For this review, take the finished solid that the model builds, in its own axes (mm). Face numbers are marked on the shaded views. A direction names the side the tool comes from. Coordinates: 2 decimals unless noted, no trailing zeros. Order: outer loops, then holes, each group sorted by start corner. A loop starts at its lowest first (then second) coordinate and runs counter-clockwise, first axis right, second up. Notation, with made-up numbers: M -2,53.5 L 30,53.5 A12 ccw 30,65.5 Z; hole C 57.5,-29 d6. An arc over 180 degrees is marked long. Use CSV: the item, a comma, the result in double quotes.
```python
from build123d import *

# Parameters (mm, degrees)
SKETCH1_W                       = 40
SKETCH1_H                       = 35
BOSS_EXTRUDE1_DEPTH             = 20
TAP_DRILL_FOR_M3X0_5_TAP1_D     = 2.5
TAP_DRILL_FOR_M3X0_5_TAP1_DEPTH = 4
F_8_4_8_4_DIAMETER_HOLE2_D      = 8.4
F_8_4_8_4_DIAMETER_HOLE2_DEPTH  = 15
F_8_4_8_4_DIAMETER_HOLE2_TIP    = 2.5236146
F_8_4_8_4_DIAMETER_HOLE1_D      = 8.4
F_8_4_8_4_DIAMETER_HOLE1_DEPTH  = 35
F_8_4_8_4_DIAMETER_HOLE1_TIP    = 2.5236146
F_7_0_7_DIAMETER_HOLE1_D        = 7
F_7_0_7_DIAMETER_HOLE1_DEPTH    = 15
F_7_0_7_DIAMETER_HOLE1_TIP      = 2.103012167
F_8_0_8_DIAMETER_HOLE1_D        = 8
F_8_0_8_DIAMETER_HOLE1_DEPTH    = 5.5
TAP_DRILL_FOR_M3X0_5_TAP2_D     = 2.5
TAP_DRILL_FOR_M3X0_5_TAP2_DEPTH = 5.5
CHAMFER1_SIZE                   = 0.5
G1_8_TAPPED_HOLE1_D             = 8.8
G1_8_TAPPED_HOLE1_DEPTH         = 10


with BuildPart() as part:
    # Sketch1 → Boss-Extrude1 (new body)
    with BuildSketch(Plane(origin=(0, 0, 0), x_dir=(1, 0, 0), z_dir=(0, 1, 0))):
        Rectangle(SKETCH1_W, SKETCH1_H)
    extrude(amount=BOSS_EXTRUDE1_DEPTH)

    # Tap Drill for M3x0.5 Tap1
    with Locations(Plane(origin=(0, 20, 0), x_dir=(1, 0, 0), z_dir=(0, 1, 0))):
        with Locations((-17, 14.5), (17, 14.5), (17, -14.5), (-17, -14.5)):
            Hole(TAP_DRILL_FOR_M3X0_5_TAP1_D / 2, depth=TAP_DRILL_FOR_M3X0_5_TAP1_DEPTH)

    # Ø8.4 (8.4) Diameter Hole2
    with Locations(Plane(origin=(0, 20, 0), x_dir=(1, 0, 0), z_dir=(0, 1, 0))):
        with Locations((-10, 0), (10, 0)):
            Hole(F_8_4_8_4_DIAMETER_HOLE2_D / 2, depth=F_8_4_8_4_DIAMETER_HOLE2_DEPTH)
            with Locations((0, 0, -(F_8_4_8_4_DIAMETER_HOLE2_DEPTH + F_8_4_8_4_DIAMETER_HOLE2_TIP / 2))):  # 118° drill point
                Cone(0, F_8_4_8_4_DIAMETER_HOLE2_D / 2, F_8_4_8_4_DIAMETER_HOLE2_TIP, mode=Mode.SUBTRACT)

    # Ø8.4 (8.4) Diameter Hole1
    with Locations(Plane.ZY.offset(20)):
        with Locations((0, 5)):
            Hole(F_8_4_8_4_DIAMETER_HOLE1_D / 2, depth=F_8_4_8_4_DIAMETER_HOLE1_DEPTH)
            with Locations((0, 0, -(F_8_4_8_4_DIAMETER_HOLE1_DEPTH + F_8_4_8_4_DIAMETER_HOLE1_TIP / 2))):  # 118° drill point
                Cone(0, F_8_4_8_4_DIAMETER_HOLE1_D / 2, F_8_4_8_4_DIAMETER_HOLE1_TIP, mode=Mode.SUBTRACT)

    # Ø7.0 (7) Diameter Hole1
    with Locations(Plane(origin=(0, 0, 0), x_dir=(-1, 0, 0), z_dir=(0, -1, 0))):
        with Locations((10, -10), (-10, -10), (-10, 10), (10, 10)):
            Hole(F_7_0_7_DIAMETER_HOLE1_D / 2, depth=F_7_0_7_DIAMETER_HOLE1_DEPTH)
            with Locations((0, 0, -(F_7_0_7_DIAMETER_HOLE1_DEPTH + F_7_0_7_DIAMETER_HOLE1_TIP / 2))):  # 118° drill point
                Cone(0, F_7_0_7_DIAMETER_HOLE1_D / 2, F_7_0_7_DIAMETER_HOLE1_TIP, mode=Mode.SUBTRACT)

    # Ø8.0 (8) Diameter Hole1
    with Locations(Plane(origin=(0, 20, 0), x_dir=(1, 0, 0), z_dir=(0, 1, 0))):
        with Locations((-10, 10), (10, 10), (10, -10), (-10, -10)):
            Hole(F_8_0_8_DIAMETER_HOLE1_D / 2, depth=F_8_0_8_DIAMETER_HOLE1_DEPTH)

    # Tap Drill for M3x0.5 Tap2
    with Locations(Plane.XY.offset(17.5)):
        with Locations((-10.622143035, 11), (-10.622143035, 3), (10.622143035, 3), (10.622143035, 11)):
            tap_drill_for_m3x0_5_tap2 = Hole(TAP_DRILL_FOR_M3X0_5_TAP2_D / 2, depth=TAP_DRILL_FOR_M3X0_5_TAP2_DEPTH)

    # Mirror1: Tap Drill for M3x0.5 Tap2 across plane
    add(tap_drill_for_m3x0_5_tap2.mirror(Plane.XY), mode=Mode.SUBTRACT)

    # Chamfer1
    chamfer1_edges = [part.edges().sort_by_distance(p)[0] for p in [
        (-20, 20, 0),
        (0, 20, 17.5),
        (20, 20, 0),
        (0, 0, 17.5),
        (-20, 0, 0),
        (0, 0, -17.5),
        (20, 0, 0),
        (0, 20, -17.5),
        (20, 10, 17.5),
        (-20, 10, 17.5),
        (-20, 10, -17.5),
        (20, 10, -17.5),
    ]]
    chamfer(chamfer1_edges, length=CHAMFER1_SIZE)

    # G1/8 Tapped Hole1
    with Locations(Plane(origin=(0, 20, 0), x_dir=(1, 0, 0), z_dir=(0, 1, 0))):
        with Locations((-10, 0), (10, 0)):
            Hole(G1_8_TAPPED_HOLE1_D / 2, depth=G1_8_TAPPED_HOLE1_DEPTH)


solid = part.part
```
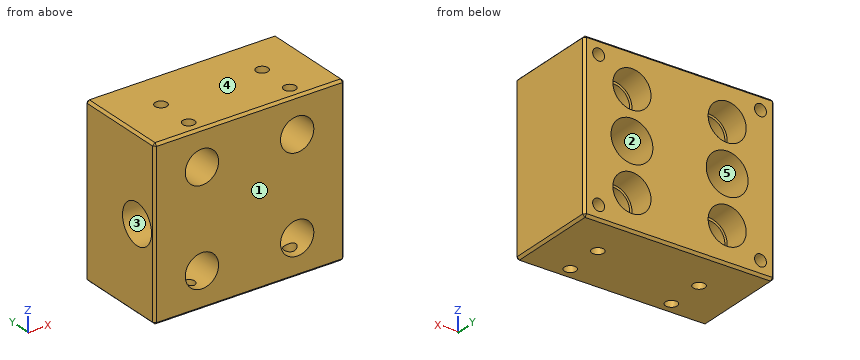
Item 1: Clearance check with flat-ended pins moving along their axes: pin 1 Ø6.5 at (x, z) = (10.5, 10.5) entering from +Y; pin 2 Ø5 at (x, z) = (10, 0) entering from -Y; pin 3 Ø2 at (x, z) = (17, 14.5) entering from +Y; pin 4 Ø2 at (x, y) = (10.62, 3) entering from +Z. State where each tip first meets the part, or that it passes through.
Solutions:
pin 1,"y = 14.5"
pin 2,"y = 0"
pin 3,"y = 16"
pin 4,"z = 6.9"
Item 2: Add section B-B on x = -13. State how many separate pieces and enclosed holes the cut face has, and give its area (3 significant figures).
Solutions:
separate pieces,"3"
enclosed holes,"0"
area,"410 mm^2"
Item 3: Draft analysis for pull direction Y (two halves, no side actions). For the marked faces 1, 2 and 3, state which applies: released by +Y, released by -Y, zero draft, split by the parting line, or undercut.
Solutions:
face 1,"released by -Y"
face 2,"zero draft"
face 3,"undercut"
Item 4: Add section D-D on z = -15. State the section outline as (x, y) points, and give its area (3 significant figures).
Solutions:
outline,"M -20,0.5 L -19.5,0 L 19.5,0 L 20,0.5 L 20,19.5 L 19.5,20 L 18.15,20 L 18.15,16 L 15.85,16 L 15.85,20 L -15.85,20 L -15.85,16 L -18.15,16 L -18.15,20 L -19.5,20 L -20,19.5 Z; hole C -10.62,3 d2.5; hole C -10.62,11 d2.5; hole C 10.62,3 d2.5; hole C 10.62,11 d2.5"
area,"762 mm^2"
Item 5: Add section C-C on x = -17. State the section outline as (y, z) points.
Solutions:
outline,"M 0,-17 L 0.5,-17.5 L 19.5,-17.5 L 20,-17 L 20,-15.75 L 16,-15.75 L 16,-13.25 L 20,-13.25 L 20,13.25 L 16,13.25 L 16,15.75 L 20,15.75 L 20,17 L 19.5,17.5 L 0.5,17.5 L 0,17 Z; hole C 5,0 d8.4"
Item 6: To check wall thickness, follow line 1 along Z through (x, y) = (-10, 8); line 2 along Z through (x, y) = (17, 18.8); line 3 along X through (y, z) = (11, -15.9). State the ranges of each line that lie inside material, in increasing order. Write a range as [from, to].
Solutions:
line 1,"[-17.5, -13.5], [-6.5, -4.2], [4.2, 6.5], [13.5, 17.5]"
line 2,"[-17.5, -15.75], [-13.25, 13.25], [15.75, 17.5]"
line 3,"[-20, -11.87], [-9.37, 9.37], [11.87, 20]"
Item 7: Add section A-A on z = -10. State the section outline as (x, y) points.
Solutions:
outline,"M -20,0.5 L -19.5,0 L -13.5,0 L -13.5,14.5 L -14,14.5 L -14,20 L -19.5,20 L -20,19.5 Z; M -6.5,0 L 6.5,0 L 6.5,14.5 L 6,14.5 L 6,20 L -6,20 L -6,14.5 L -6.5,14.5 Z; M 13.5,0 L 19.5,0 L 20,0.5 L 20,19.5 L 19.5,20 L 14,20 L 14,14.5 L 13.5,14.5 Z"
Item 8: For the marked faces 4 and 5, list the 3-axis set-ups (+Z, -Z, +X, -X, +Y, -Y) from which the entire face can be reached by the end or side of a thin tool; tool diameter is ignored.
Solutions:
face 4,"+Z, +X, -X, +Y, -Y"
face 5,"+Y"
